from build123d import *

# Parameters (mm, degrees)
F1_DEPTH  = 38.1
F3_DEPTH  = 18.796
F4_R      = 15.875
F5_DEPTH  = 18.796
F6_R      = 3.6195
F7_DEPTH  = 24.257
F9_DEPTH  = 18.796
F11_DEPTH = 19.05


with BuildPart() as f1:
    # F0 (on Top) → F1 (new body)
    with BuildSketch(Plane.XY):
        Polygon((-12.0983748909, -20.955), (12.0983748909, -20.955), (24.1967497817, 0), (12.0983748909, 20.955), (-12.0983748909, 20.955), (-24.1967497817, 0), align=None)
    extrude(amount=F1_DEPTH)

    # F2 (on face) → F3 (cut)
    with BuildSketch(Plane.XY.offset(38.1)):
        Polygon((-11.365140049, -19.685), (11.365140049, -19.685), (22.730280098, 0), (11.365140049, 19.685), (-11.365140049, 19.685), (-22.730280098, 0), align=None)
    extrude(amount=-F3_DEPTH, mode=Mode.SUBTRACT)

    # F4 (on face) → F5 (join)
    with BuildSketch(Plane.XY.offset(38.1)):
        Polygon((-22.730280098, 0), (-11.365140049, -19.685), (11.365140049, -19.685), (22.730280098, 0), (11.365140049, 19.685), (-11.365140049, 19.685), align=None)
        Circle(F4_R, mode=Mode.SUBTRACT)
    extrude(amount=-F5_DEPTH)

    # F6 (on face) → F7 (cut)
    with BuildSketch(Plane.XY.offset(38.1)):
        Circle(F6_R)
    extrude(amount=-F7_DEPTH, mode=Mode.SUBTRACT)

    # F8 (on face) → F9 (join)
    with BuildSketch(Plane(origin=(0, 0, 0), x_dir=(1, 0, 0), z_dir=(0, 0, -1))):
        Polygon((-2.286, 20.955), (0, 20.955), (0, 23.241), (-3.429, 23.241), align=None)
        Polygon((0, 23.241), (0, 20.955), (2.286, 20.955), (3.429, 23.241), align=None)
    extrude(amount=-F9_DEPTH)

    # F10 (on face) → F11 (cut)
    with BuildSketch(Plane(origin=(0, 0, 0), x_dir=(1, 0, 0), z_dir=(0, 0, -1))):
        Polygon((19.4175623363, 8.2777954744), (18.1475623363, 10.4775), (15.9478578107, 9.2075), (17.8528578107, 5.9079432116), align=None)
        Polygon((15.9478578107, 9.2075), (18.1475623363, 10.4775), (16.8775623363, 12.6772045256), (14.0428578107, 12.5070567884), align=None)
    extrude(amount=-F11_DEPTH, mode=Mode.SUBTRACT)


solid = f1.part
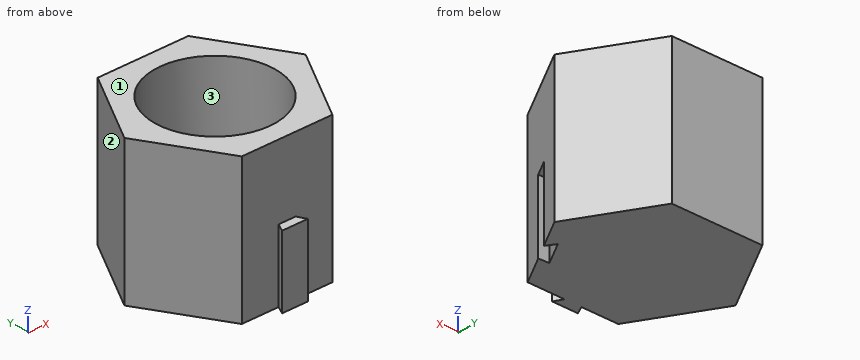
Build history of the part. All positions in model axes, mm. Face numbers are marked on the shaded views. Give positions to 0.01 mm unless a question says otherwise; leave off trailing zeros. Order: outer loops, then holes, each group sorted by start corner. A loop starts at its lowest first (then second) coordinate and runs counter-clockwise, first axis right, second up. Notation, with made-up numbers: M -21.5,16.25 L 10.5,16.25 A26 ccw 10.5,40.25 Z; hole C 46.25,-20.5 d8. An arc over 180 degrees is marked long. Use one line per item in the form item = value.
1) Saw through at B-B (x = 0). Give the cut face in (y, z) (1 decimal), plus the area to 3 significant figures.
Calculated:
outline = M -23.2,0 L 21,0 L 21,38.1 L 15.9,38.1 L 15.9,19.3 L 3.6,19.3 L 3.6,13.8 L -3.6,13.8 L -3.6,19.3 L -15.9,19.3 L -15.9,38.1 L -21,38.1 L -21,18.8 L -23.2,18.8 Z
area = 1,000 mm2
2) Saw through at C-C (y = 13). Give the cut face in (x, z).
Calculated:
outline = M -16.69,0 L 16.69,0 L 16.69,38.1 L 9.11,38.1 L 9.11,19.3 L -9.11,19.3 L -9.11,38.1 L -16.69,38.1 Z
3) Drop flat-ended pins along their axis: pin 1 (4 mm diameter, centred on y = 5.5, z = 15.5, fed in from +X); pin 2 (3.5 mm diameter, centred on x = -0.5, y = -0.5, fed in from +Z); pin 3 (5 mm diameter, centred on x = 0, y = 7, fed in from +Z). Give the stop position or say it passes through.
Calculated:
pin_1 = 22.18
pin_2 = 13.84
pin_3 = 19.3
4) Probe probe 1 along Y at (x, z) = (0, 24) (3 decimals); probe 2 along Y at (x, z) = (0, 17) (1 decimal); probe 3 along Z at (x, y) = (-5, 7). List the from-to ranges inside material, lowest first.
Calculated:
probe_1 = -20.955 to -15.875, 15.875 to 20.955
probe_2 = -23.2 to -3.6, 3.6 to 21
probe_3 = 0 to 19.3
5) Saw through at D-D (z = 11). Give the cut face in (x, y) (3 decimals), plus the area to 3 significant figures.
Calculated:
outline = M -24.197,0 L -12.098,-20.955 L -2.286,-20.955 L -3.429,-23.241 L 3.429,-23.241 L 2.286,-20.955 L 12.098,-20.955 L 16.878,-12.677 L 14.043,-12.507 L 17.853,-5.908 L 19.418,-8.278 L 24.197,0 L 12.098,20.955 L -12.098,20.955 Z
area = 1,520 mm2
6) Saw through at A-A (z = 25.5). Give the cut face in (x, y) (3 decimals).
Calculated:
outline = M -24.197,0 L -12.098,-20.955 L 12.098,-20.955 L 24.197,0 L 12.098,20.955 L -12.098,20.955 Z; hole C 0,0 d31.75
7) Two-plate mould, pull along X, no slides. Class the marked faces 1, 2 and 3: released by +X, released by -X, zero draft, split by the parting line, or undercut.
Calculated:
face_1 = zero draft
face_2 = released by -X
face_3 = undercut
